Here's how the part is built. I have some questions about the finished solid (model axes, mm). Coordinates: 2 decimals unless noted, no trailing zeros. Write each loop counter-clockwise with the first axis right and the second up, starting at its lowest first coordinate (ties: lowest second). Pieces come first, ordered by that corner, then holes. Notation, with made-up numbers: (31.25, -15) -> (90.25, -15) arc R21 cw to (90.25, 12) -> close; hole circle Ø5 at (26, 87.25). An arc over 180 degrees is marked (long way). Answer in a Markdown table with one row per item. Add a question column.
from build123d import *

# Parameters (mm, degrees)
F1_DEPTH      = 50
F1_DEPTH_BACK = 5
F3_DEPTH      = 25.001
F3_DEPTH_BACK = 25.001
F4_R          = 2


with BuildPart() as f1:
    # F0 (on Front) → F1 (new body, two sides)
    with BuildSketch(Plane.XZ) as f1_sk:
        with BuildLine():
            ThreePointArc((14.5, 22.5), (7.3569694848, 24.3704230117), (0, 25))
            ThreePointArc((0, 25), (-7.3569694848, 24.3704230117), (-14.5, 22.5))
            ThreePointArc((-14.5, 22.5), (-19.4027296199, 19.4027296199), (-22.5, 14.5))
            ThreePointArc((-22.5, 14.5), (-24.3704230117, 7.3569694848), (-25, 0))
            ThreePointArc((-25, 0), (-24.3704230117, -7.3569694848), (-22.5, -14.5))
            ThreePointArc((-22.5, -14.5), (-19.4027296199, -19.4027296199), (-14.5, -22.5))
            ThreePointArc((-14.5, -22.5), (-7.3569694848, -24.3704230117), (0, -25))
            ThreePointArc((0, -25), (7.3569694848, -24.3704230117), (14.5, -22.5))
            ThreePointArc((14.5, -22.5), (19.4027296199, -19.4027296199), (22.5, -14.5))
            ThreePointArc((22.5, -14.5), (24.3704230117, -7.3569694848), (25, 0))
            ThreePointArc((25, 0), (24.3704230117, 7.3569694848), (22.5, 14.5))
            ThreePointArc((22.5, 14.5), (19.4027296199, 19.4027296199), (14.5, 22.5))
        make_face()
    extrude(amount=-F1_DEPTH)
    extrude(f1_sk.sketch, amount=F1_DEPTH_BACK)

    # F2 (on Top) → F3 (cut, two sides)
    with BuildSketch(Plane.XY) as f3_sk:
        Polygon((-25, 25), (0, 0), (25, 25), (25, 50), (0, 50), (-25, 50), align=None)
    extrude(amount=-F3_DEPTH, mode=Mode.SUBTRACT)
    extrude(f3_sk.sketch, amount=F3_DEPTH_BACK, mode=Mode.SUBTRACT)

    # F4
    f4_edges = [f1.edges().sort_by_distance(p)[0] for p in [
        (0, 0, 0),
    ]]
    fillet(f4_edges, radius=F4_R)


solid = f1.part
Q1. If we mould it in two halves opening along X, with no side actions, what happens to faces 1 (the cylindrical face through (-19.46, 5.887, -19.345)), 2 (the flat face through (-13, 13, 0)), 3 (the flat face through (13, 13, 0)), 4 (the cylindrical face through (0.2, 0.6, 25))? For each: pulls with the +X half, pulls with the -X half, needs draft (parallel to the pull), parting line crosses it, or undercut.
Q2. Imagine slicing it at D-D on x = 4. Please give me the cut outline in (y, z), plus the area to 3 significant figures.
Q3. I need wall thicknesses on line 1 (X direction, y = 2.5, z = 9.5) (3 decimals); line 2 (X direction, y = 11.5, z = -2.5); line 3 (Y direction, x = 18, z = 19.5). Which ranges of each line are inside material? Lowest first, please. Write a range as [from, to].
Q4. Imagine slicing it at C-C on y = 19. Please give me the cut outline in (x, z), plus the area to 3 significant figures.
Q5. I'm going to push flat-ended pins straight in: P1, Ø4, axis at x = -13.5, y = 5.5, coming from the +Z side; P2, Ø10, axis at x = -16.5, y = 5.5, coming from the -Z side; P3, Ø3, axis at y = 7.5, z = -19.5, coming from the +X side. Where does each tip first touch, or does it pass through?
Q6. Imagine slicing it at A-A on y = 11.5. Please give me the cut outline in (x, z), plus the area to 3 significant figures.
Q7. Imagine slicing it at B-B on z = -11.5. Please give me the cut outline in (x, y), plus the area to 3 significant figures.
Result sheet:
| question | item | result |
|---|---|---|
| 1 | face 1 | pulls with the -X half |
| 1 | face 2 | undercut |
| 1 | face 3 | undercut |
| 1 | face 4 | parting line crosses it |
| 2 | outline | (-5, -24.81) -> (4, -24.81) -> (4, 24.81) -> (-5, 24.81) -> close |
| 2 | area | 447 mm^2 |
| 3 | line 1 | x = [-23.945, -2.5], [2.5, 23.945] |
| 3 | line 2 | x = [-24.93, -11.5], [11.5, 24.93] |
| 3 | line 3 | y = [-5, 18] |
| 4 | outline | (-22.5, -14.5) arc R13.17 ccw to (-19, -19.79) -> (-19, 19.79) arc R13.17 ccw to (-22.5, 14.5) arc R43.3 ccw to start; (19, -19.79) arc R13.17 ccw to (22.5, -14.5) arc R43.3 ccw to (22.5, 14.5) arc R13.17 ccw to (19, 19.79) -> close |
| 4 | area | 344 mm^2 |
| 5 | P1 | stops at z = 23.44 |
| 5 | P2 | stops at z = -23.44 |
| 5 | P3 | stops at x = 20.62 |
| 6 | outline | (-22.5, -14.5) arc R13.17 ccw to (-14.5, -22.5) arc R43.3 ccw to (-11.5, -23.44) -> (-11.5, 23.44) arc R43.3 ccw to (-14.5, 22.5) arc R13.17 ccw to (-22.5, 14.5) arc R43.3 ccw to start; (11.5, -23.44) arc R43.3 ccw to (14.5, -22.5) arc R13.17 ccw to (22.5, -14.5) arc R43.3 ccw to (22.5, 14.5) arc R13.17 ccw to (14.5, 22.5) arc R43.3 ccw to (11.5, 23.44) -> close |
| 6 | area | 1,000 mm^2 |
| 7 | outline | (-23.44, -5) -> (23.44, -5) -> (23.44, 23.44) -> (1.41, 1.41) arc R2 cw to (-1.41, 1.41) -> (-23.44, 23.44) -> close |
| 7 | area | 785 mm^2 |
